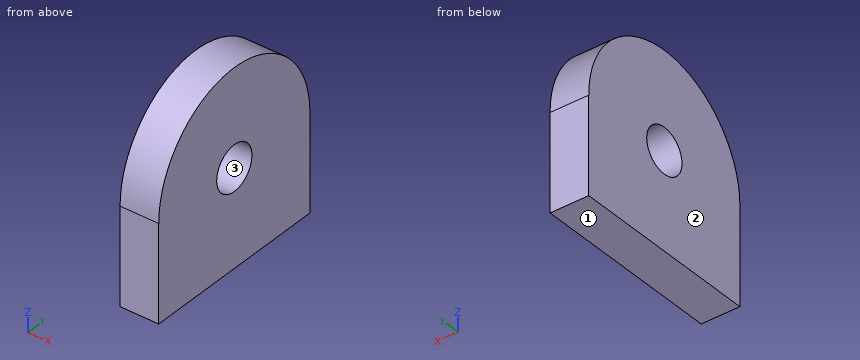
Autodesk Inventor part; units mm, degrees
ref_plane "YZ Plane" through (0, 0, 0) normal (1, 0, 0) x (0, 1, 0)
ref_plane "XZ Plane" through (0, 0, 0) normal (0, 1, 0) x (-1, 0, 0)
ref_plane "XY Plane" through (0, 0, 0) normal (0, 0, 1) x (1, 0, 0)
sketch "Sketch1" plane through (0, 0, 0) normal (0, 0, 1) x (1, 0, 0)
  line L0 (7.5, 7.5) -> (-7.5, 7.5)
  line L1 (-7.5, -7.5) -> (7.5, -7.5)
  line L2 (-1.5, 7.5) -> (1.5, 7.5)
  line L3 (1.5, 7.5) -> (1.5, -7.5)
  line L4 (1.5, -7.5) -> (-1.5, -7.5)
  line L5 (-1.5, -7.5) -> (-1.5, 7.5)
  line L6 (-1.5, 7.5) -> (1.5, -7.5) construction
  line L7 (1.5, 7.5) -> (-1.5, -7.5) construction
  point P0 (0, 0)
  dimension "d0" = 3
extrude "Extrusion1" add sketch "Sketch1" along normal blind 15
sketch "Sketch2" plane through (1.5, -7.5, 0) normal (1, 0, 0) x (0, 0, -1)
  line L0 (0, 15) -> (0, 0)
  line L1 (0, 15) -> (-15, 15)
  line L2 (-15, 0) -> (-15, 15)
  line L3 (-15, 15) -> (-7.5, 15)
  line L4 (0, 15) -> (-15, 15)
  line L5 (0, 0) -> (-15, 0)
  line L6 (0, 0) -> (-15, 0)
  arc A0 (-7.5, 15) -> (-7.5, 0) centre (-7.5, 7.5) ccw
  line L7 (-15, 15) -> (-15, 0)
  circle A1 centre (-7.5, 7.5) radius 1.75
  point P0 (0, 7.5)
  point P1 (-10, 7.5)
  dimension "d3" = 7.5
  dimension "d7" = 3.5
extrude "Extrusion2" cut sketch "Sketch2" against normal up to next contours A0 L2 L1 | L5 L2 A0 | A1
properties part number "weight_holder_string_loop"
CAD build for the part. Positions are in the model's coordinates, mm. Face numbers are marked on the shaded views. Round coordinates to 2 decimals unless told otherwise and drop trailing zeros. Order: outer loops, then holes, each group sorted by start corner. A loop starts at its lowest first (then second) coordinate and runs counter-clockwise, first axis right, second up. Notation, with made-up numbers: (-20, 82) - (14, 82) arc R17 cw to (14, 90) - close; hole circle Ø11 at (-21.75, 84). An arc over 180 degrees is marked (long way). Return JSON: item names as keys, results as strings.
(1) Cut at B-B (z = 8.5). Give the cut face in (x, y).
Answer key:
{"outline": "(-1.5, -7.43) - (1.5, -7.43) - (1.5, -1.44) - (-1.5, -1.44) - close; (-1.5, 1.44) - (1.5, 1.44) - (1.5, 7.43) - (-1.5, 7.43) - close"}
(2) Cut at A-A (y = 0). Give the cut face in (x, z), then the cut area to 3 significant figures.
Answer key:
{"outline": "(-1.5, 0) - (1.5, 0) - (1.5, 5.75) - (-1.5, 5.75) - close; (-1.5, 9.25) - (1.5, 9.25) - (1.5, 15) - (-1.5, 15) - close", "area": "34.5 mm^2"}
(3) Pin check, flat tip, straight feed: pin 1 Ø3 at (y, z) = (0, 7.5) entering from -X. Stop position of the tip, or through.
Answer key:
{"pin 1": "passes through"}
(4) Pull direction Z, two halves, no side cores. Call the marked faces 1, 2 and 3: +Z half, -Z half, draft (parallel to the pull), parting line (faces both ways), or undercut.
Answer key:
{"face 1": "-Z half", "face 2": "draft", "face 3": "undercut"}
(5) Cut at D-D (y = -6.5). Give the cut face in (x, z).
Answer key:
{"outline": "(-1.5, 0) - (1.5, 0) - (1.5, 11.24) - (-1.5, 11.24) - close"}
(6) Cut at C-C (x = 0.7). Give the cut face in (y, z).
Answer key:
{"outline": "(-7.5, 0) - (7.5, 0) - (7.5, 7.5) arc R7.5 ccw to (-7.5, 7.5) - close; hole circle Ø3.5 at (0, 7.5)"}
(7) Wall check: probe 1 along Y at (x, z) = (-0.3, 7.5); probe 2 along Y at (x, z) = (-0.55, 12.25); probe 3 along Z at (x, y) = (-0.2, -2). Give the ranges that are in metal, low to high. Write a range as from..to.
Answer key:
{"probe 1": "y = -7.5..-1.75, 1.75..7.5", "probe 2": "y = -5.8..5.8", "probe 3": "z = 0..14.73"}
